Here's how the part is built. I have some questions about the finished solid (model axes, mm). A direction names the side the tool comes from. Coordinates: 2 decimals unless noted, no trailing zeros. Order: outer loops, then holes, each group sorted by start corner. A loop starts at its lowest first (then second) coordinate and runs counter-clockwise, first axis right, second up. Notation, with made-up numbers: (15.25, -37.5) - (74.25, -37.5) arc R34 ccw to (74.25, -0.5) - close; hole circle Ø4 at (85, 48.25). An arc over 180 degrees is marked (long way). Answer in a Markdown table with one row per item. Add a question column.
Item 1: If I drill on line 1 along Z through (x, y) = (0, 245); line 2 along Z through (x, y) = (260, -209); line 3 along X through (y, z) = (-398, -208), over which ranges is the centre line in solid material (lowest first)? Write a range as from..to.
Item 2: On a 3-axis mill with a long thin cutter (end or side, diameter ignored), from which of +Z, -Z, +X, -X, +Y, -Y can I reach the whole of each face in a straight line? I mean faces 1 (the cylindrical face through (-42.99, -8.89, 327.39)), 2 (the flat face through (-77, 38.1, -324)), 3 (the flat face through (-77, -38.1, -324)). Say none if no direction works.
Item 3: I want a section at A-A (x = 0). Please give me the cut outline in (y, z) (3 decimals).
Item 4: Will these pins go through, and if not, where does the flat tip stop? pin 1 Ø12 at (x, y) = (236, -305.5) entering from -Z; pin 2 Ø1 at (x, y) = (110.5, -405.5) entering from -Z; pin 3 Ø6 at (x, y) = (-259, 292) entering from +Z.
Item 5: I want a section at B-B (z = 35). Please give me the cut outline in (x, y) (3 decimals).
Item 6: I want a section at D-D (y = 150). Please give me the cut outline in (x, z).
Item 7: Thinking about a two-plate mould opening in X: for faces 4 (the cylindrical face through (-42.159, 8.89, 321.094)), 5 (the cylindrical face through (-7.47, -0.533, -339.643)), 6 (the flat face through (243, 635, -219)), which applies, +X half, -X half, draft (parallel to the pull), parting line (faces both ways), or undercut?
Item 8: I want a section at C-C (z = -129.5). Please give me the cut outline in (x, y), plus the area to 3 significant figures.
```python
from build123d import *

# Parameters (mm, degrees)
F1_DEPTH = 38.1
F2_R     = 17.4625
F3_DEPTH = 679.451
F4_R     = 330.2
F4_R_2   = 323.85
F5_DEPTH = 635


with BuildPart() as f1:
    # F0 (on Front) → F1 (new body, symmetric)
    with BuildSketch(Plane.XZ):
        with BuildLine():
            ThreePointArc((330.2, 0), (0, -330.2), (-330.2, 0))
            Line((-330.2, 0), (-330.2, 398.4625))
            Line((-330.2, 398.4625), (-339.725, 398.4625))
            Line((-339.725, 398.4625), (-339.725, 0))
            ThreePointArc((-339.725, 0), (0, -339.725), (339.725, 0))
            Line((339.725, 0), (339.725, 398.4625))
            Line((339.725, 398.4625), (330.2, 398.4625))
            Line((330.2, 398.4625), (330.2, 0))
        make_face()
    extrude(amount=F1_DEPTH, both=True)

    # F2 (on face) → F3 (cut, through all)
    with BuildSketch(Plane(origin=(-339.725, 0, 0), x_dir=(0, -1, 0), z_dir=(-1, 0, 0))):
        with Locations((0, 363.5375)):
            Circle(F2_R)
    extrude(amount=-F3_DEPTH, mode=Mode.SUBTRACT)

    # F4 (on Front) → F5 (join, symmetric)
    with BuildSketch(Plane.XZ):
        Circle(F4_R)
        Circle(F4_R_2, mode=Mode.SUBTRACT)
    extrude(amount=F5_DEPTH, both=True)


solid = f1.part
```
Values follow:
| question | item | result |
|---|---|---|
| 1 | line 1 | z = -330.2..-323.85, 323.85..330.2 |
| 1 | line 2 | z = -203.55..-193.08, 193.08..203.55 |
| 1 | line 3 | x = -256.45..-248.22, 248.22..256.45 |
| 2 | face 1 | none |
| 2 | face 2 | -Z, +Y |
| 2 | face 3 | -Z, -Y |
| 3 | outline | (-635, -330.2) - (-38.1, -330.2) - (-38.1, -339.725) - (38.1, -339.725) - (38.1, -330.2) - (635, -330.2) - (635, -323.85) - (-635, -323.85) - close; (-635, 323.85) - (635, 323.85) - (635, 330.2) - (-635, 330.2) - close |
| 4 | pin 1 | stops at z = -236.92 |
| 4 | pin 2 | stops at z = -311.34 |
| 4 | pin 3 | stops at z = 208.56 |
| 5 | outline | (-339.725, -38.1) - (-330.2, -38.1) - (-330.2, 38.1) - (-339.725, 38.1) - close; (-328.34, -635) - (-321.953, -635) - (-321.953, 635) - (-328.34, 635) - close; (321.953, -635) - (328.34, -635) - (328.34, 635) - (321.953, 635) - close; (330.2, -38.1) - (339.725, -38.1) - (339.725, 38.1) - (330.2, 38.1) - close |
| 6 | outline | circle Ø660.4 at (0, 0); hole circle Ø647.7 at (0, 0) |
| 7 | face 4 | undercut |
| 7 | face 5 | parting line |
| 7 | face 6 | draft |
| 8 | outline | (-314.07, -38.1) - (-303.75, -38.1) - (-303.75, -635) - (-296.83, -635) - (-296.83, 635) - (-303.75, 635) - (-303.75, 38.1) - (-314.07, 38.1) - close; (296.83, -635) - (303.75, -635) - (303.75, -38.1) - (314.07, -38.1) - (314.07, 38.1) - (303.75, 38.1) - (303.75, 635) - (296.83, 635) - close |
| 8 | area | 19,100 mm^2 |
